Source: CAD feature listing. Evaluate the final solid. Frame: model axes, mm. A direction names the side the tool comes from. Round coordinates to 2 decimals unless told otherwise and drop trailing zeros. Loops run counter-clockwise (first coordinate to the right, second up) from the corner with the lowest first, then second, coordinate; pieces in that order, holes last. Notation, with made-up numbers: (52.25, 28.5) - (79.25, 28.5) arc R14 cw to (79.25, 35.5) - close; hole circle Ø2 at (37, 54.5). An arc over 180 degrees is marked (long way). One line per question, with ' | ' between items.
from build123d import *

# Parameters (mm, degrees)
EXTRUDE_1_DEPTH     = 5.33
SKETCH_1_W          = 0.5
SKETCH_1_H          = 0.5
EXTRUDE_2_DEPTH     = 2.54
SKETCH_1_2_W        = 0.5
SKETCH_1_2_H        = 0.5
EXTRUDE_3_DEPTH     = 10.16
SKETCH_4_R          = 0.2
CUT_EXTRUDE_1_DEPTH = 0.5
SKETCH_5_W          = 9.7
SKETCH_5_H          = 0.5
EXTRUDE_4_DEPTH     = 1.27
SKETCH_6_W          = 9.7
SKETCH_6_H          = 0.5
EXTRUDE_5_DEPTH     = 1.27
SKETCH_7_W          = 0.5
SKETCH_7_H          = 9.7
EXTRUDE_6_DEPTH     = 2.54
SKETCH_8_W          = 1.372733762
SKETCH_8_H          = 9.815585296
CUT_EXTRUDE_2_DEPTH = 2.54
SKETCH_9_W          = 9.522444549
SKETCH_9_H          = 3.637804143
CUT_EXTRUDE_3_DEPTH = 1
FILLET_1_R          = 1
FILLET_2_R          = 1.5
SKETCH_10_W         = 0.5
SKETCH_10_H         = 0.5
CUT_EXTRUDE_4_DEPTH = 5
SKETCH_11_R         = 0.1469903
CUT_EXTRUDE_5_DEPTH = 2


with BuildPart() as part:
    # Эскиз3 → Вытянуть1 (new body)
    with BuildSketch(Plane.XY.offset(2.54)):
        with BuildLine():
            Line((-0.325, -1.53), (3.105, -1.53))
            Line((3.105, -1.53), (3.99, 0))
            ThreePointArc((3.99, 0), (3.240904038, 1.868477631), (1.39, 2.66))
            ThreePointArc((1.39, 2.66), (-0.460904038, 1.868477631), (-1.21, 0))
            Line((-1.21, 0), (-0.325, -1.53))
        make_face()
    extrude(amount=EXTRUDE_1_DEPTH)

    # Эскиз1 → Вытянуть2 (add)
    with BuildSketch(Plane.XY):
        with Locations((1.39, 0)):
            Rectangle(SKETCH_1_W, SKETCH_1_H)
        Rectangle(SKETCH_1_W, SKETCH_1_H)
        with Locations((2.78, 0)):
            Rectangle(SKETCH_1_W, SKETCH_1_H)
    extrude(amount=EXTRUDE_2_DEPTH)

    # Эскиз1<2> → Вытянуть3 (add)
    with BuildSketch(Plane.XY):
        with Locations((1.39, 0)):
            Rectangle(SKETCH_1_2_W, SKETCH_1_2_H)
        Rectangle(SKETCH_1_2_W, SKETCH_1_2_H)
        with Locations((2.78, 0)):
            Rectangle(SKETCH_1_2_W, SKETCH_1_2_H)
    extrude(amount=-EXTRUDE_3_DEPTH)

    # Эскиз4 → Вырез-Вытянуть1 (cut)
    with BuildSketch(Plane.XY.offset(7.87)):
        Circle(SKETCH_4_R)
    extrude(amount=-CUT_EXTRUDE_1_DEPTH, mode=Mode.SUBTRACT)

    # Эскиз5 → Вытянуть4 (add)
    with BuildSketch(Plane(origin=(3.03, 0, 0), x_dir=(0, 0, -1), z_dir=(1, 0, 0))):
        with Locations((5.31, 0)):
            Rectangle(SKETCH_5_W, SKETCH_5_H)
    extrude(amount=EXTRUDE_4_DEPTH)

    # Эскиз6 → Вытянуть5 (add)
    with BuildSketch(Plane.ZY.offset(0.25)):
        with Locations((-5.31, 0)):
            Rectangle(SKETCH_6_W, SKETCH_6_H)
    extrude(amount=EXTRUDE_5_DEPTH)

    # Эскиз7 → Вытянуть6 (add)
    with BuildSketch(Plane(origin=(0, -0.25, 0), x_dir=(1, 0, 0), z_dir=(0, 1, 0))):
        with Locations((1.39, 5.31)):
            Rectangle(SKETCH_7_W, SKETCH_7_H)
    extrude(amount=-EXTRUDE_6_DEPTH)

    # Эскиз8 → Вырез-Вытянуть2 (cut)
    with BuildSketch(Plane.XZ.offset(0.25)):
        with Locations((-0.333633119, -5.867792648)):
            Rectangle(SKETCH_8_W, SKETCH_8_H)
        with Locations((3.113633119, -5.867792648)):
            Rectangle(SKETCH_8_W, SKETCH_8_H)
    extrude(amount=-CUT_EXTRUDE_2_DEPTH, mode=Mode.SUBTRACT)

    # Эскиз9 → Вырез-Вытянуть3 (cut)
    with BuildSketch(Plane(origin=(1.64, 0, 0), x_dir=(0, 0, -1), z_dir=(1, 0, 0))):
        with Locations((5.721222275, -0.471097928)):
            Rectangle(SKETCH_9_W, SKETCH_9_H)
    extrude(amount=-CUT_EXTRUDE_3_DEPTH, mode=Mode.SUBTRACT)

    # Скругление1
    fillet_1_edges = [part.edges().sort_by_distance(p)[0] for p in [
        (-1.02, 0, -0.96),
        (1.39, -2.29, -0.96),
        (3.8, 0, -0.96),
        (3.03, 0, -0.46),
        (1.39, -0.25, -0.46),
        (-0.25, 0, -0.46),
    ]]
    fillet(fillet_1_edges, radius=FILLET_1_R)

    # Скругление2
    fillet_2_edges = [part.edges().sort_by_distance(p)[0] for p in [
        (-1.52, 0, -0.46),
        (1.39, -2.79, -0.46),
        (4.3, 0, -0.46),
        (0.25, 0, -0.96),
        (1.39, 0.25, -0.96),
        (2.53, 0, -0.96),
    ]]
    fillet(fillet_2_edges, radius=FILLET_2_R)

    # Эскиз10 → Вырез-Вытянуть4 (cut)
    with BuildSketch(Plane(origin=(0, 0, -10.16), x_dir=(-1, 0, 0), z_dir=(0, 0, -1))):
        with Locations((-1.39, -2.54)):
            Rectangle(SKETCH_10_W, SKETCH_10_H)
        with Locations((1.27, 0)):
            Rectangle(SKETCH_10_W, SKETCH_10_H)
        with Locations((-4.05, 0)):
            Rectangle(SKETCH_10_W, SKETCH_10_H)
    extrude(amount=-CUT_EXTRUDE_4_DEPTH, mode=Mode.SUBTRACT)

    # Эскиз11 → Вырез-Вытянуть5 (cut)
    with BuildSketch(Plane(origin=(0, 0, -5.16), x_dir=(-1, 0, 0), z_dir=(0, 0, -1))):
        with Locations((-1.39, -2.54)):
            Circle(SKETCH_11_R)
    extrude(amount=-CUT_EXTRUDE_5_DEPTH, mode=Mode.SUBTRACT)


solid = part.part
1. Contact query for flat-ended pins moving along their axis: P1, Ø1.5, axis at y = -0.5, z = 0.5, coming from the -X side; P2, Ø0.6, axis at y = 0, z = 1, coming from the +X side; P3, Ø0.6, axis at x = 1.5, z = -4, coming from the +Y side. Output: stop coordinate, or through.
Worked out:
P1: stops at x = -0.59 | P2: stops at x = 3.03 | P3: stops at y = -2.29
2. Section query B-B, the plane z = 0.75. Return loops of the section in (x, y), plus the area to 3 significant figures.
Worked out:
outline: (-0.25, -0.25) - (0.25, -0.25) - (0.25, 0.25) - (-0.25, 0.25) - close; (1.14, -0.25) - (1.64, -0.25) - (1.64, 0.25) - (1.14, 0.25) - close; (2.53, -0.25) - (3.03, -0.25) - (3.03, 0.25) - (2.53, 0.25) - close | area: 0.750 mm2
3. Section query C-C, the plane z = 4.75. Return loops of the section in (x, y) (3 decimals).
Worked out:
outline: (-1.21, 0) - (-0.325, -1.53) - (3.105, -1.53) - (3.99, 0) arc R2.63 ccw to (1.39, 2.66) arc R2.63 ccw to start
4. Access query for faces 5 (the flat face through (3.5, 0.25, -1)), 6 (the flat face through (3.5, -0.25, -1)), 7 (the flat face through (1.64, -2, -1)), 8 (the cylindrical face through (1.39, -0.18, -0.51)), 9 (the flat face through (-1, -0.25, -1)). Directions: +Z, -Z, +X, -X, +Y, -Y. A direction counts if a zero-diameter tool reaches every point of the face in a straight line with its end or side. Return the directions, or none.
Worked out:
face 5: -Z, +X, -X, +Y | face 6: -Z, +X, -Y | face 7: -Z, +Y, -Y | face 8: -Z, +Y | face 9: -Z, -X, -Y
5. Material intervals for probe 1 along X at (y, z) = (-0.1, 0.75); probe 2 along Z at (x, y) = (-0.25, -1.05); probe 3 along X at (y, z) = (1.45, 3), sorted ascending.
Worked out:
probe 1: x = -0.25 to 0.25, 1.14 to 1.64, 2.53 to 3.03 | probe 2: z = 2.54 to 7.87 | probe 3: x = -0.79 to 3.57
6. Section query D-D, the plane y = -2.54. Return loops of the section in (x, z).
Worked out:
outline: (1.14, -5.16) - (1.24, -5.16) - (1.24, -3.16) - (1.54, -3.16) - (1.54, -5.16) - (1.64, -5.16) - (1.64, -1.13) - (1.14, -1.13) - close
7. Mould query, pull axis X, two halves, no side actions, for faces 1 (the flat face through (1.14, -2, -1)), 2 (the flat face through (3.54, -0.78, 5.17)), 3 (the cylindrical face through (-0.44, 1.89, 5.17)), 4 (the flat face through (-1, 0.25, -1)). Classes: released by +X, released by -X, zero draft, split by the parting line, or undercut.
Worked out:
face 1: undercut | face 2: released by +X | face 3: released by -X | face 4: zero draft
8. Section query A-A, the plane z = -4. Return loops of the section in (x, y).
Worked out:
outline: (-1.52, -0.25) - (-1.02, -0.25) - (-1.02, 0.25) - (-1.52, 0.25) - close; (1.14, -2.79) - (1.64, -2.79) - (1.64, -2.29) - (1.14, -2.29) - close; (3.8, -0.25) - (4.3, -0.25) - (4.3, 0.25) - (3.8, 0.25) - close; hole circle Ø0.29 at (1.39, -2.54)
